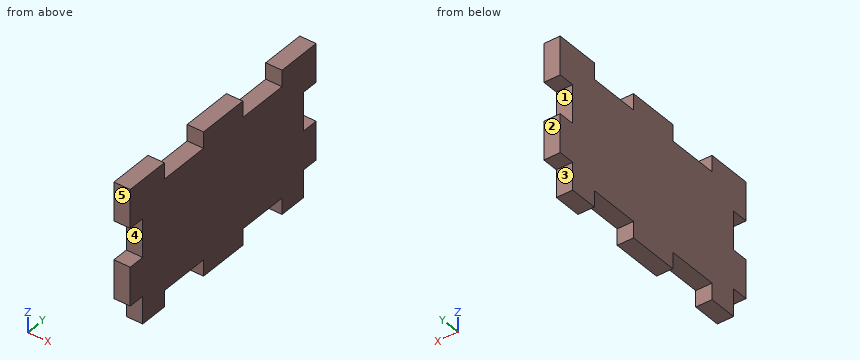
```python
from build123d import *

# Parameters (mm, degrees)
SKETCH1_W           = 35.35
SKETCH1_H           = 47.35
BOSS_EXTRUDE1_DEPTH = 3.175
SKETCH2_W           = 7.5
SKETCH2_H           = 47.35
CUT_EXTRUDE1_DEPTH  = 4.175
SKETCH3_W           = 3.175
SKETCH3_H           = 10
SKETCH3_W_2         = 7.5
SKETCH3_H_2         = 3.175
SKETCH3_W_3         = 5.35
CUT_EXTRUDE2_DEPTH  = 4.175


with BuildPart() as part:
    # Sketch1 → Boss-Extrude1 (new body)
    with BuildSketch(Plane(origin=(0, 0, 0), x_dir=(0, 0, -1), z_dir=(1, 0, 0))):
        with Locations((17.675, 23.675)):
            Rectangle(SKETCH1_W, SKETCH1_H)
    extrude(amount=BOSS_EXTRUDE1_DEPTH)

    # Sketch2 → Cut-Extrude1 (cut, through all)
    with BuildSketch(Plane.ZY):
        with Locations((-31.6, 23.675)):
            Rectangle(SKETCH2_W, SKETCH2_H)
    extrude(amount=-CUT_EXTRUDE1_DEPTH, mode=Mode.SUBTRACT)

    # Sketch3 → Cut-Extrude2 (cut, through all)
    with BuildSketch(Plane.ZY):
        with Locations((-1.5875, 13.675)):
            Rectangle(SKETCH3_W, SKETCH3_H)
        with Locations((-1.5875, 33.675)):
            Rectangle(SKETCH3_W, SKETCH3_H)
        with Locations((-26.2625, 13.675)):
            Rectangle(SKETCH3_W, SKETCH3_H)
        with Locations((-26.2625, 33.675)):
            Rectangle(SKETCH3_W, SKETCH3_H)
        with Locations((-11.25, 45.7625)):
            Rectangle(SKETCH3_W_2, SKETCH3_H_2)
        with Locations((-11.25, 1.5875)):
            Rectangle(SKETCH3_W_2, SKETCH3_H_2)
        with Locations((-25.175, 45.7625)):
            Rectangle(SKETCH3_W_3, SKETCH3_H_2)
        with Locations((-25.175, 1.5875)):
            Rectangle(SKETCH3_W_3, SKETCH3_H_2)
    extrude(amount=-CUT_EXTRUDE2_DEPTH, mode=Mode.SUBTRACT)


solid = part.part
```
Input: part model. Units: mm. Frame: model coordinates. Face numbers are marked on the shaded views. A direction names the side the tool comes from. Give positions to 0.01 mm unless a question says otherwise; leave off trailing zeros. Loops run counter-clockwise (first coordinate to the right, second up) from the corner with the lowest first, then second, coordinate; pieces in that order, holes last. Notation, with made-up numbers: M 1.25,-9 L 8.25,-9 A25 ccw 8.25,29 Z; hole C -6.5,-30 d1. An arc over 180 degrees is marked long. Answer as CSV lines item,"result". Start each with the question number.
1. Pin query (flat end, axial travel): P1, Ø1.6, axis at x = 2, y = 1, coming from the -Z side; P2, Ø1, axis at x = 1, y = 12.5, coming from the -Z side (3 decimals); P3, Ø1.6, axis at x = 2, y = 36, coming from the +Z side (3 decimals). Return the tip coordinate at first contact, or that it passes through.
2. Reachability of the marked faces 3, 4 and 5 from +Z, -Z, +X, -X, +Y, -Y: full face, straight path, thin tool, end or side. Return the list, or none.
3. Line query: L1, parallel to Y at x = 1.5, z = -24.75 (3 decimals); L2, parallel to Z at x = 0.55, y = 2; L3, parallel to Z at x = 2.4, y = 33 (3 decimals). Output: solid intervals per line, ascending.
4. Pull-direction query (Z, two-part tool) for the marked faces 1 and 2; classes: released by +Z, released by -Z, zero draft, split by the parting line, or undercut.
5. Section B-B on z = -10. Return loops of the section in (x, y) (3 decimals).
6. Section C-C on y = 13. Return loops of the section in (x, z) (3 decimals).
Computed values:
1,P1,"stops at z = -22.5"
1,P2,"stops at z = -24.675"
1,P3,"stops at z = -3.175"
2,face 3,"-Z, +X, -X, +Y"
2,face 4,"+X, -X, -Y"
2,face 5,"+Z, -Z, +X, -X, -Y"
3,L1,"y = 3.175 to 8.675, 18.675 to 28.675, 38.675 to 44.175"
3,L2,"z = -22.5 to -15, -7.5 to 0"
3,L3,"z = -24.675 to -3.175"
4,face 1,"undercut"
4,face 2,"zero draft"
5,outline,"M 0,3.175 L 3.175,3.175 L 3.175,44.175 L 0,44.175 Z"
6,outline,"M 0,-24.675 L 3.175,-24.675 L 3.175,-3.175 L 0,-3.175 Z"
